Autodesk Inventor part; units mm, degrees
ref_plane "Work Plane1" through (30.1625, 0, 0) normal (0, 0, -1) x (1, 0, 0)
ref_plane "YZ Plane" through (0, 0, 0) normal (1, 0, 0) x (0, 1, 0)
ref_plane "XZ Plane" through (0, 0, 0) normal (0, 1, 0) x (-1, 0, 0)
sketch "Sketch1" plane through (0, 0, 0) normal (0, 0, 1) x (1, 0, 0)
  line L0 (-3.3, 0) -> (10, 0)
  line L1 (10, 0) -> (10, 2.5)
  line L2 (10, 2.5) -> (1.6, 2.5)
  line L3 (1.6, 2.5) -> (1.1091, 2.2835)
  line L4 (1.1091, 2.2835) -> (0, 2.2835)
  line L5 (0, 2.2835) -> (0, 4.25)
  line L6 (-5.96, 0) -> (12.66, 0)
  line L7 (0, -0.85) -> (0, 5.1)
  line L8 (-3.3, 0) -> (-3.3, 3.9613)
  line L9 (0, 4.25) -> (-3.3, 3.9613)
  line L10 (1.6, 2.5) -> (0, 2.5) construction
  dimension "d0" = 10
  dimension "d1" = 8.4
  dimension "d2" = 0.4909
  dimension "d3" = 3.3
  dimension "d4" = 5
  dimension "d5" = 4.567
  dimension "d9" = 8.5
  dimension "d10" = 5
revolve "Body" add sketch "Sketch1" angle 360 about axis through (-3.3, 0, 0) along (1, 0, 0)
sketch "Sketch2" plane through (-3.3, 0, 0) normal (-1, 0, 0) x (0, 0, 1)
  circle A0 centre (0, 0) radius 4.25
  line L0 (0, 0) -> (0, 3.9613)
  line L1 (-4.25, 0.6) -> (4.25, 0.6)
  line L2 (4.25, 0.6) -> (4.25, -0.6)
  line L3 (4.25, -0.6) -> (-4.25, -0.6)
  line L4 (-4.25, -0.6) -> (-4.25, 0.6)
  line L5 (-4.25, 0) -> (4.25, 0) construction
  line L6 (0, 0.6) -> (0, -0.6) construction
  point P0 (0, 0)
  dimension "d11" = 1.2
  dimension "d12" = 8.5
fillet "Fillet1" radius 0.2 1 edges at (-3.3, -3.9613, 0)
extrude "Slot" cut sketch "Sketch2" against normal blind 1.3 contours A0 L3 L1 | L2 L3 A0 | A0 L1 L2 | A0 L4 L1 | L3 L4 A0
thread "Thread"
chamfer "Chamfer1" distance 0.433 distance2 0.4909 1 edges at (10, -2.5, 0) measured on face at (10, 0.6684, -0.7339)
ref_plane "Work Plane1" through (30.1625, 0, 0) normal (0, 0, -1) x (1, 0, 0)
equation "\"d11\" = SBR"
equation "\"d12\" = KOD"
equation "\"d14\" = RR"
equation "\"d19\" = STI"
equation "\"d15\" = GEL"
equation "\"d17\" = -0.5 * SPD + 0.5 * GD"
equation "\"d0\" = NLG"
equation "\"d1\" = GEL"
equation "\"d3\" = KOH"
equation "\"d4\" = GD"
equation "\"d5\" = BDM"
equation "\"d9\" = KOD"
equation "\"d10\" = KEWI"
equation "\"GD\" = 5"
equation "\"NLG\" = 10"
equation "\"GEL\" = 8.4"
equation "\"KOD\" = 8.5"
equation "\"KOH\" = 3.3"
equation "\"GAL\" = 0.61345 * PTC"
equation "\"SPD\" = 4.13397"
equation "\"BDM\" = 4.56699"
equation "\"GUL\" = 0.61345 * PTC"
equation "\"RR\" = 0.2"
equation "\"SBR\" = 1.2"
equation "\"STI\" = 1.3"
equation "\"KEWI\" = 5deg"
equation "\"PTC\" = 0.8"
equation "\"THREADDIA\" = 5"
equation "\"TOA\" = 30deg"
equation "\"NND\" = 5"
equation "\"GD1\" = THREADDIA - 1.2269 * PTC"
properties part number "DIN 84 - M5 x 10" material "Steel, Mild"
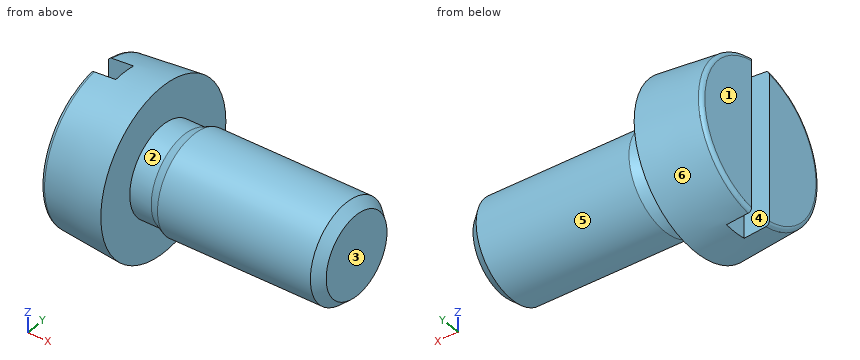
Source: CAD feature listing. Evaluate the final solid. Frame: model axes, mm. Face numbers are marked on the shaded views. A direction names the side the tool comes from. Give positions to 0.01 mm unless a question says otherwise; leave off trailing zeros. Loops run counter-clockwise (first coordinate to the right, second up) from the corner with the lowest first, then second, coordinate; pieces in that order, holes last. Notation, with made-up numbers: (68.25, 56.5) - (123.25, 56.5) arc R38 cw to (123.25, 94.5) - close; hole circle Ø11 at (-40, 32). An arc over 180 degrees is marked (long way). Use CSV: the item, a comma, the result in double quotes. Start each with the question number.
1. Ray query, L1, parallel to X at y = 0.5, z = 2.5; L2, parallel to X at y = 2.5, z = 1.25; L3, parallel to Z at x = 1.5, y = 1. Return the intervals inside material, ascending.
2. Draft query along X for the marked faces 1, 2, 3 and 4. Return one class per face: +X half, -X half, draft (parallel to the pull), parting line (faces both ways), or undercut.
3. Reachability of the marked faces 5 and 6 from +Z, -Z, +X, -X, +Y, -Y: full face, straight path, thin tool, end or side. Return the list, or none.
4. Section A-A (y = 0). Output: boundary loops of the cut face in (x, z).
5. Section B-B (z = 0). Output: boundary loops of the cut face in (x, y), then the cut area to 3 significant figures.
6. Section C-C (x = 4). Output: boundary loops of the cut face in (y, z), then the cut area to 3 significant figures.
7. Pin query (flat end, axial travel): pin 1 (1 mm diameter, centred on x = -2.5, z = 0, fed in from -Y); pin 2 (3 mm diameter, centred on x = 6, z = -1.5, fed in from +Y). Return the tip coordinate at first contact, or that it passes through.
Response:
1,L1,"-2 to 0"
1,L2,"-3.3 to 0"
1,L3,"-2.24 to 2.24"
2,face 1,"-X half"
2,face 2,"undercut"
2,face 3,"+X half"
2,face 4,"draft"
3,face 5,"+X"
3,face 6,"-X"
4,outline,"(-2, -4.08) - (0, -4.25) - (0, -2.28) - (1.11, -2.28) - (1.6, -2.5) - (9.51, -2.5) - (10, -2.07) - (10, 2.07) - (9.51, 2.5) - (1.6, 2.5) - (1.11, 2.28) - (0, 2.28) - (0, 4.25) - (-2, 4.08) - close"
5,outline,"(-3.3, -3.78) arc R0.2 ccw to (-3.12, -3.98) - (0, -4.25) - (0, -2.28) - (1.11, -2.28) - (1.6, -2.5) - (9.51, -2.5) - (10, -2.07) - (10, 2.07) - (9.51, 2.5) - (1.6, 2.5) - (1.11, 2.28) - (0, 2.28) - (0, 4.25) - (-3.12, 3.98) arc R0.2 ccw to (-3.3, 3.78) - (-3.3, 0.6) - (-2, 0.6) - (-2, -0.6) - (-3.3, -0.6) - close"
5,area,"74.7 mm²"
6,outline,"circle Ø5 at (0, 0)"
6,area,"19.6 mm²"
7,pin 1,"y = -4.08"
7,pin 2,"y = 2.5"
